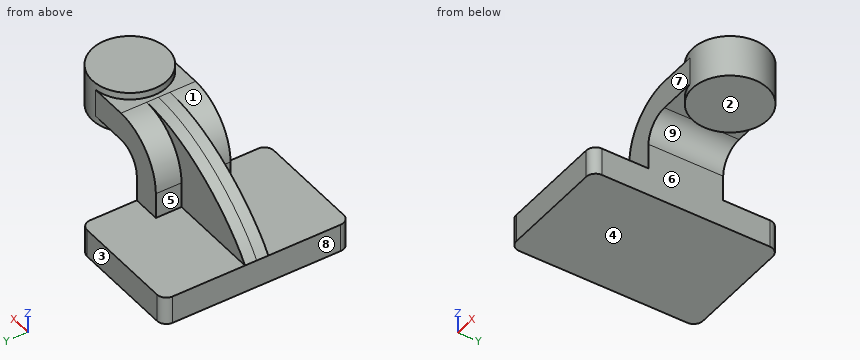
```python
from build123d import *

# Parameters (mm, degrees)
F1_DEPTH = 63.5
F2_DEPTH = 7.9375
F3_DEPTH = 25.4
F0_W     = 25.2419677258
F0_H     = 19.05
F4_DEPTH = 25.4
F6_R     = 6.35


# Not quite as in the source:
# - a feature names something its author has since deleted; it is built from what else it names


with BuildPart() as f1:
    # F0 (on Front) → F1 (new body, symmetric)
    with BuildSketch(Plane.XZ):
        Polygon((-41.275, 9.525), (-41.275, -9.525), (41.275, -9.525), (41.275, 9.525), (22.225, 9.525), align=None)
    extrude(amount=F1_DEPTH, both=True)

    # F0 (on Front) → F2 (join, symmetric)
    with BuildSketch(Plane.XZ):
        with BuildLine():
            add(Edge.make_bspline(
                [(-41.275, 9.525), (-28.5215713084, 29.158225283), (12.6376561821, 62.4269843102), (57.15, 61.9252)],
                knots=[0, 0, 0, 0, 111.5045361635, 111.5045361635, 111.5045361635, 111.5045361635], degree=3))
            Line((-41.275, 9.525), (22.225, 9.525))
            Line((22.225, 9.525), (22.225, 27.0002))
            ThreePointArc((22.225, 27.0002), (32.4542956671, 51.6959043329), (57.15, 61.9252))
        make_face()
    extrude(amount=F2_DEPTH, both=True)

    # F0 (on Front) → F3 (join, symmetric)
    with BuildSketch(Plane.XZ):
        with BuildLine():
            Line((22.225, 9.525), (41.275, 9.525))
            Line((41.275, 9.525), (41.275, 27.0002))
            ThreePointArc((41.275, 27.0002), (45.9246798487, 38.2255201513), (57.15, 42.8752))
            Line((57.15, 42.8752), (60.325, 42.8752))
            Line((60.325, 42.8752), (60.325, 61.9252))
            Line((60.325, 61.9252), (57.15, 61.9252))
            ThreePointArc((57.15, 61.9252), (32.4542956671, 51.6959043329), (22.225, 27.0002))
            Line((22.225, 27.0002), (22.225, 9.525))
        make_face()
    extrude(amount=F3_DEPTH, both=True)

    # F0 (on Front) → F4 (join, symmetric)
    with BuildSketch(Plane.XZ):
        with Locations((72.9459838629, 52.4002)):
            Rectangle(F0_W, F0_H)
    extrude(amount=F4_DEPTH, both=True)

    # F0 (on Front) → F5 (revolve)
    with BuildSketch(Plane.XZ):
        Polygon((85.5669677258, 66.675), (85.5669677258, 61.9252), (85.5669677258, 42.8752), (85.5669677258, 38.1), (111.125, 38.1), (111.125, 66.675), align=None)
    revolve(axis=Axis((85.5669677258, 0, 52.3875), (0, 0, -1)))

    # F6
    f6_edges = [f1.edges().sort_by_distance(p)[0] for p in [
        (-41.275, -63.5, 0),
        (41.275, -63.5, 0),
        (41.275, 63.5, 0),
        (-41.275, 63.5, 0),
    ]]
    fillet(f6_edges, radius=F6_R)


solid = f1.part
```
Could you check a few things on this model? Use its own coordinates, in mm. Face numbers are marked on the shaded views. A direction names the side the tool comes from. Coordinates: 2 decimals unless noted, no trailing zeros. Loops run counter-clockwise (first coordinate to the right, second up) from the corner with the lowest first, then second, coordinate; pieces in that order, holes last.
1) Please list where these lines run through material, in increasing order: line 1 along Y through (x, z) = (36, 15); line 2 along Z through (x, y) = (-1, -11) (3 decimals); line 3 along X through (y, z) = (19, 5.5) (3 decimals).
Reported:
line 1: y = -25.4 to 25.4
line 2: z = -9.525 to 9.525
line 3: x = -41.275 to 41.275
2) Thinking about a two-plate mould opening in X: for the marked faces 6, 7, 8 and 9, which applies, released by +X, released by -X, zero draft, split by the parting line, or undercut?
Reported:
face 6: released by +X
face 7: zero draft
face 8: released by -X
face 9: undercut
3) Will these pins go through, and if not, where does the flat tip stop? pin 1 Ø15.5 at (x, z) = (-11.5, 25.5) entering from -Y; pin 2 Ø2 at (x, y) = (-1, -10) entering from +Z (3 decimals); pin 3 Ø12 at (y, z) = (16, 34) entering from -X.
Reported:
pin 1: stops at y = -7.94
pin 2: stops at z = 9.525
pin 3: stops at x = 22.24
4) Imagine slicing it at A-A (z = -1). List the corners of the cut face in (x, y) for me (3 decimals), and give its area (3 significant figures).
Reported:
outline: (-41.275, -57.15) arc R6.35 ccw to (-34.925, -63.5) - (34.925, -63.5) arc R6.35 ccw to (41.275, -57.15) - (41.275, 57.15) arc R6.35 ccw to (34.925, 63.5) - (-34.925, 63.5) arc R6.35 ccw to (-41.275, 57.15) - close
area: 10,400 mm2
5) Imagine slicing it at C-C (x = 73). List the corners of the cut face in (y, z) for me (3 decimals).
Reported:
outline: (-25.4, 42.875) - (-22.255, 42.875) - (-22.255, 38.1) - (22.255, 38.1) - (22.255, 42.875) - (25.4, 42.875) - (25.4, 61.925) - (22.255, 61.925) - (22.255, 66.675) - (-22.255, 66.675) - (-22.255, 61.925) - (-25.4, 61.925) - close
6) Imagine slicing it at D-D (y = 36). List the corners of the cut face in (x, z) for me (3 decimals).
Reported:
outline: (-41.275, -9.525) - (41.275, -9.525) - (41.275, 9.525) - (-41.275, 9.525) - close
7) Which directions (+Z, -Z, +X, -X, +Y, -Y) give clear straight access to the entire face, cutting with the end or side of a thin tool? Please do the marked faces 1, 2, 3, 4 and 5.
Reported:
face 1: +Z, -X, -Y
face 2: -Z, +X, +Y, -Y
face 3: +Z, -Z, +X, -X, +Y
face 4: -Z, +X, -X, +Y, -Y
face 5: +Z, -X, +Y
